Input: part model. Units: mm. Frame: model coordinates. A direction names the side the tool comes from. Give positions to 0.01 mm unless a question says otherwise; leave off trailing zeros. Order: outer loops, then holes, each group sorted by start corner. A loop starts at its lowest first (then second) coordinate and runs counter-clockwise, first axis right, second up. Notation, with made-up numbers: (79.5, 69.25) - (93.5, 69.25) arc R24 ccw to (93.5, 93.25) - close; hole circle Ø8 at (50, 14.5). An arc over 180 degrees is marked (long way). Answer in a Markdown table with one row per item. Add a question column.
from build123d import *
from OCP.BRepFilletAPI import BRepFilletAPI_MakeChamfer

# Parameters (mm, degrees)
SKETCH1_W           = 65
SKETCH1_H           = 100
BOSS_EXTRUDE1_DEPTH = 2
SKETCH2_W           = 65
SKETCH2_H           = 100
SKETCH2_W_2         = 57
SKETCH2_H_2         = 92
BOSS_EXTRUDE2_DEPTH = 3
FILLET1_R           = 5
BOSS_EXTRUDE3_DEPTH = 10
SKETCH6_R           = 18
BOSS_EXTRUDE4_DEPTH = 5
CHAMFER1_SIZE       = 10
SKETCH7_R           = 13
CUT_EXTRUDE1_DEPTH  = 80.726093596
BOSS_EXTRUDE6_DEPTH = 2
BOSS_EXTRUDE7_DEPTH = 7
CHAMFER2_SIZE       = 1.3
CHAMFER2_SIZE2      = 4.000988598


with BuildPart() as part:
    # Sketch1 → Boss-Extrude1 (new body)
    with BuildSketch(Plane(origin=(0, 0, 0), x_dir=(1, 0, 0), z_dir=(0, 1, 0))):
        with Locations((0, -20)):
            Rectangle(SKETCH1_W, SKETCH1_H)
    extrude(amount=BOSS_EXTRUDE1_DEPTH)

    # Sketch2 → Boss-Extrude2 (add)
    with BuildSketch(Plane(origin=(0, 2, 0), x_dir=(1, 0, 0), z_dir=(0, 1, 0))):
        with Locations((0, -20)):
            Rectangle(SKETCH2_W, SKETCH2_H)
        with Locations((0, -20)):
            Rectangle(SKETCH2_W_2, SKETCH2_H_2, mode=Mode.SUBTRACT)
    extrude(amount=BOSS_EXTRUDE2_DEPTH)

    # Fillet1
    fillet1_edges = [part.edges().sort_by_distance(p)[0] for p in [
        (-28.5, 3.5, 66),
        (28.5, 3.5, 66),
        (28.5, 3.5, -26),
        (-28.5, 3.5, -26),
        (-32.5, 2.5, -30),
        (32.5, 2.5, -30),
        (32.5, 2.5, 70),
        (-32.5, 2.5, 70),
    ]]
    fillet(fillet1_edges, radius=FILLET1_R)

    # Sketch4 → Boss-Extrude3 (add)
    with BuildSketch(Plane(origin=(0, 5, 0), x_dir=(1, 0, 0), z_dir=(0, 1, 0))):
        with BuildLine():
            Line((-32.5, 25), (-32.5, -65))
            ThreePointArc((-32.5, -65), (-31.035533906, -68.535533906), (-27.5, -70))
            Line((-27.5, -70), (27.5, -70))
            ThreePointArc((27.5, -70), (31.035533906, -68.535533906), (32.5, -65))
            Line((32.5, -65), (32.5, 25))
            ThreePointArc((32.5, 25), (31.035533906, 28.535533906), (27.5, 30))
            Line((27.5, 30), (-27.5, 30))
            ThreePointArc((-27.5, 30), (-31.035533906, 28.535533906), (-32.5, 25))
        make_face()
        with BuildLine():
            Line((-30.5, 25), (-30.5, -65))
            ThreePointArc((-30.5, -65), (-29.621320344, -67.121320344), (-27.5, -68))
            Line((-27.5, -68), (27.5, -68))
            ThreePointArc((27.5, -68), (29.621320344, -67.121320344), (30.5, -65))
            Line((30.5, -65), (30.5, 25))
            ThreePointArc((30.5, 25), (29.621320344, 27.121320344), (27.5, 28))
            Line((27.5, 28), (-27.5, 28))
            ThreePointArc((-27.5, 28), (-29.621320344, 27.121320344), (-30.5, 25))
        make_face(mode=Mode.SUBTRACT)
    extrude(amount=BOSS_EXTRUDE3_DEPTH)

    # Sketch6 → Boss-Extrude4 (add)
    with BuildSketch(Plane(origin=(0, -5, 0), x_dir=(-1, 0, 0), z_dir=(0, -1, 0))):
        with Locations(Location((0, 0, 0), (0, 0, 90))):
            Circle(SKETCH6_R)
    extrude(amount=-BOSS_EXTRUDE4_DEPTH)

    # Chamfer1
    # the kernel refuses this chamfer: 10 mm, written as the material it adds along each edge
    with BuildSketch(Plane(origin=(0, 0, 0), x_dir=(0, 0, -1), z_dir=(-1, 0, 0))) as chamfer1_piece_1_section:
        Polygon((18 + CHAMFER1_SIZE, 0), (18, CHAMFER1_SIZE), (18, 0), align=None)
    chamfer1_piece_1 = revolve(axis=Axis((0, 0, 0), (0, -1, 0)), mode=Mode.PRIVATE)
    chamfer1_piece_1 = split(chamfer1_piece_1, bisect_by=Plane(origin=(0, -5, 25.515578953), z_dir=(0, 1, 0)), keep=Keep.TOP, mode=Mode.PRIVATE)
    add(chamfer1_piece_1)

    # Sketch7 → Cut-Extrude1 (cut, through all)
    with BuildSketch(Plane.XZ.offset(5)):
        with Locations(Location((0, 0, 0), (0, 0, 270))):
            Circle(SKETCH7_R)
    extrude(amount=-CUT_EXTRUDE1_DEPTH, mode=Mode.SUBTRACT)

    # Sketch8 → Boss-Extrude6 (add)
    with BuildSketch(Plane(origin=(0, -5, 0), x_dir=(-1, 0, 0), z_dir=(0, -1, 0))):
        with BuildLine():
            ThreePointArc((-8.942785339, 7.230255208), (-4.172190868, 10.71647439), (1.699808228, 11.373682429))
            Line((1.699808228, 11.373682429), (1.921522345, 12.857206224))
            ThreePointArc((1.921522345, 12.857206224), (-4.716389677, 12.114275398), (-10.109235601, 8.173331975))
            Line((-10.109235601, 8.173331975), (-8.942785339, 7.230255208))
        make_face()
        with BuildLine():
            Line((1.921522345, 12.857206224), (1.699808228, 11.373682429))
            ThreePointArc((1.699808228, 11.373682429), (4.307975824, 10.662614328), (6.678083991, 9.362328461))
            Line((6.678083991, 9.362328461), (7.549138424, 10.583501739))
            ThreePointArc((7.549138424, 10.583501739), (4.869885714, 12.053390109), (1.921522345, 12.857206224))
        make_face()
        with BuildLine():
            Line((12.464656553, 3.692199481), (11.026426951, 3.266176464))
            ThreePointArc((11.026426951, 3.266176464), (11.380990948, 1.650165153), (11.5, 0))
            ThreePointArc((11.5, 0), (10.443646499, -4.814586982), (7.468652556, -8.744668604))
            Line((7.468652556, -8.744668604), (8.442824628, -9.885277553))
            ThreePointArc((8.442824628, -9.885277553), (11.80586126, -5.442576588), (13, 0))
            ThreePointArc((13, 0), (12.865468029, 1.865404086), (12.464656553, 3.692199481))
        make_face()
        with BuildLine():
            ThreePointArc((7.468652556, -8.744668604), (6.263348903, -9.644711531), (4.950877613, -10.37973077))
            Line((4.950877613, -10.37973077), (5.596644259, -11.733608697))
            ThreePointArc((5.596644259, -11.733608697), (7.080307455, -10.902717383), (8.442824628, -9.885277553))
            Line((8.442824628, -9.885277553), (7.468652556, -8.744668604))
        make_face()
        with BuildLine():
            ThreePointArc((-8.359560208, 6.758716825), (-3.900091464, 10.017573887), (1.58895117, 10.631920531))
            Line((1.58895117, 10.631920531), (1.699808228, 11.373682429))
            ThreePointArc((1.699808228, 11.373682429), (-4.172190868, 10.71647439), (-8.942785339, 7.230255208))
            Line((-8.942785339, 7.230255208), (-8.359560208, 6.758716825))
        make_face()
        with BuildLine():
            Line((11.026426951, 3.266176464), (10.30731215, 3.053164956))
            ThreePointArc((10.30731215, 3.053164956), (10.638752408, 1.542545686), (10.75, 0))
            ThreePointArc((10.75, 0), (9.762539119, -4.500592179), (6.98156652, -8.17436413))
            Line((6.98156652, -8.17436413), (7.468652556, -8.744668604))
            ThreePointArc((7.468652556, -8.744668604), (10.443646499, -4.814586982), (11.5, 0))
            ThreePointArc((11.5, 0), (11.380990948, 1.650165153), (11.026426951, 3.266176464))
        make_face()
        with BuildLine():
            Line((-2.48051694, -12.761153385), (-2.194303447, -11.28871261))
            ThreePointArc((-2.194303447, -11.28871261), (-7.98857126, -8.272407704), (-11.205255745, -2.586937125))
            Line((-11.205255745, -2.586937125), (-12.666810842, -2.924363706))
            ThreePointArc((-12.666810842, -2.924363706), (-9.030558816, -9.351417404), (-2.48051694, -12.761153385))
        make_face()
        with BuildLine():
            Line((-2.194303447, -11.28871261), (-2.0511967, -10.552492222))
            ThreePointArc((-2.0511967, -10.552492222), (-7.467577482, -7.732902854), (-10.474478196, -2.418223834))
            Line((-10.474478196, -2.418223834), (-11.205255745, -2.586937125))
            ThreePointArc((-11.205255745, -2.586937125), (-7.98857126, -8.272407704), (-2.194303447, -11.28871261))
        make_face()
        with BuildLine():
            ThreePointArc((-11.205255745, -2.586937125), (-11.42607634, -1.301836958), (-11.5, 0))
            Line((-11.5, 0), (-13, 0))
            ThreePointArc((-13, 0), (-12.916434124, -1.471641779), (-12.666810842, -2.924363706))
            Line((-12.666810842, -2.924363706), (-11.205255745, -2.586937125))
        make_face()
    extrude(amount=-BOSS_EXTRUDE6_DEPTH)

    # Sketch8<5> → Boss-Extrude7 (add)
    with BuildSketch(Plane(origin=(0, -5, 0), x_dir=(-1, 0, 0), z_dir=(0, -1, 0))):
        with BuildLine():
            Line((1.921522345, 12.857206224), (1.699808228, 11.373682429))
            ThreePointArc((1.699808228, 11.373682429), (4.307975824, 10.662614328), (6.678083991, 9.362328461))
            Line((6.678083991, 9.362328461), (7.549138424, 10.583501739))
            ThreePointArc((7.549138424, 10.583501739), (4.869885714, 12.053390109), (1.921522345, 12.857206224))
        make_face()
        with BuildLine():
            ThreePointArc((7.468652556, -8.744668604), (6.263348903, -9.644711531), (4.950877613, -10.37973077))
            Line((4.950877613, -10.37973077), (5.596644259, -11.733608697))
            ThreePointArc((5.596644259, -11.733608697), (7.080307455, -10.902717383), (8.442824628, -9.885277553))
            Line((8.442824628, -9.885277553), (7.468652556, -8.744668604))
        make_face()
        with BuildLine():
            ThreePointArc((-11.205255745, -2.586937125), (-11.42607634, -1.301836958), (-11.5, 0))
            Line((-11.5, 0), (-13, 0))
            ThreePointArc((-13, 0), (-12.916434124, -1.471641779), (-12.666810842, -2.924363706))
            Line((-12.666810842, -2.924363706), (-11.205255745, -2.586937125))
        make_face()
    extrude(amount=-BOSS_EXTRUDE7_DEPTH)

    # Chamfer2: one chamfer whose edges measure the first distance from different faces: ONE call of the kernel's chamfer builder (chamfer() names one face for all edges)
    chamfer2_edges_1 = [part.edges().sort_by_distance(p)[0] for p in [
        (9.234397905, -3, -7.4660244),
    ]]
    chamfer2_side_1 = [part.faces().sort_by_distance(p)[0] for p in [
        (9.234397905, -4, -7.4660244),
    ]]
    chamfer2_edges_2 = [part.edges().sort_by_distance(p)[0] for p in [
        (-11.385984352, -3, -3.372682218),
    ]]
    chamfer2_side_2 = [part.faces().sort_by_distance(p)[0] for p in [
        (-11.385984352, -4, -3.372682218),
    ]]
    chamfer2_edges_3 = [part.edges().sort_by_distance(p)[0] for p in [
        (2.26585682, -3, 11.656822803),
    ]]
    chamfer2_side_3 = [part.faces().sort_by_distance(p)[0] for p in [
        (2.26585682, -4, 11.656822803),
    ]]
    chamfer2 = BRepFilletAPI_MakeChamfer(part.part.solid().wrapped)
    for e in chamfer2_edges_1:
        chamfer2.Add(CHAMFER2_SIZE, CHAMFER2_SIZE2, e.wrapped, chamfer2_side_1[0].wrapped)  # the first distance lies on this face
    for e in chamfer2_edges_2:
        chamfer2.Add(CHAMFER2_SIZE, CHAMFER2_SIZE2, e.wrapped, chamfer2_side_2[0].wrapped)  # the first distance lies on this face
    for e in chamfer2_edges_3:
        chamfer2.Add(CHAMFER2_SIZE, CHAMFER2_SIZE2, e.wrapped, chamfer2_side_3[0].wrapped)  # the first distance lies on this face
    add(Compound.cast(chamfer2.Shape()), mode=Mode.REPLACE)


solid = part.part
Q1. Contact query for flat-ended pins moving along their axis: P1, Ø1.1, axis at x = 2, z = -11.5, coming from the +Y side; P2, Ø3, axis at x = -26, z = 47, coming from the -Y side; P3, Ø2, axis at x = 9.5, z = 8.5, coming from the +Y side. Output: stop coordinate, or through.
Q2. Section C-C, the plane z = 39.5. Return loops of the section in (x, y).
Q3. Line query: probe 1 along X at (y, z) = (6.75, -14.5); probe 2 along Z at (x, y) = (-11, 5.25); probe 3 along X at (y, z) = (4, 17.5). Output: solid intervals per line, ascending.
Q4. Section A-A, the plane x = 0. Return loops of the section in (y, z).
Q5. Access query for faces 1 (the flat face through (0, 3, 66)), 2 (the cylindrical face through (-4.27, -1.55, -10.68)), 3 (the conical face through (6.981, -4.757, -22.169)). Directions: +Z, -Z, +X, -X, +Y, -Y. A direction counts if a zero-diameter tool reaches every point of the face in a straight line with its end or side. Return the directions, or none.
Q6. Section B-B, the plane y = 12. Return loops of the section in (x, z).
Q7. Section D-D, the plane y = 3.5. Return loops of the section in (x, z).
Computed:
| question | item | result |
|---|---|---|
| 1 | P1 | stops at y = -3 |
| 1 | P2 | stops at y = 0 |
| 1 | P3 | stops at y = 2 |
| 2 | outline | (-32.5, 0) - (32.5, 0) - (32.5, 15) - (30.5, 15) - (30.5, 5) - (28.5, 5) - (28.5, 2) - (-28.5, 2) - (-28.5, 5) - (-30.5, 5) - (-30.5, 15) - (-32.5, 15) - close |
| 3 | probe 1 | x = -32.5 to -30.5, 30.5 to 32.5 |
| 3 | probe 2 | z = -30 to -28, 68 to 70 |
| 3 | probe 3 | x = -32.5 to -28.5, 28.5 to 32.5 |
| 4 | outline | (-5, -23) - (0, -28) - (0, -30) - (15, -30) - (15, -28) - (5, -28) - (5, -26) - (2, -26) - (2, -13) - (-3, -13) - (-3, -10.75) - (-5, -10.75) - close; (-5, 13) - (2, 13) - (2, 66) - (5, 66) - (5, 68) - (15, 68) - (15, 70) - (0, 70) - (0, 28) - (-5, 23) - close |
| 5 | face 1 | +Y |
| 5 | face 2 | +Y, -Y |
| 5 | face 3 | -Y |
| 6 | outline | (-32.5, -25) arc R5 ccw to (-27.5, -30) - (27.5, -30) arc R5 ccw to (32.5, -25) - (32.5, 65) arc R5 ccw to (27.5, 70) - (-27.5, 70) arc R5 ccw to (-32.5, 65) - close; hole (-30.5, -25) arc R3 ccw to (-27.5, -28) - (27.5, -28) arc R3 ccw to (30.5, -25) - (30.5, 65) arc R3 ccw to (27.5, 68) - (-27.5, 68) arc R3 ccw to (-30.5, 65) - close |
| 7 | outline | (-32.5, -25) arc R5 ccw to (-27.5, -30) - (27.5, -30) arc R5 ccw to (32.5, -25) - (32.5, 65) arc R5 ccw to (27.5, 70) - (-27.5, 70) arc R5 ccw to (-32.5, 65) - close; hole (-28.5, -21) arc R5 ccw to (-23.5, -26) - (23.5, -26) arc R5 ccw to (28.5, -21) - (28.5, 61) arc R5 ccw to (23.5, 66) - (-23.5, 66) arc R5 ccw to (-28.5, 61) - close |
